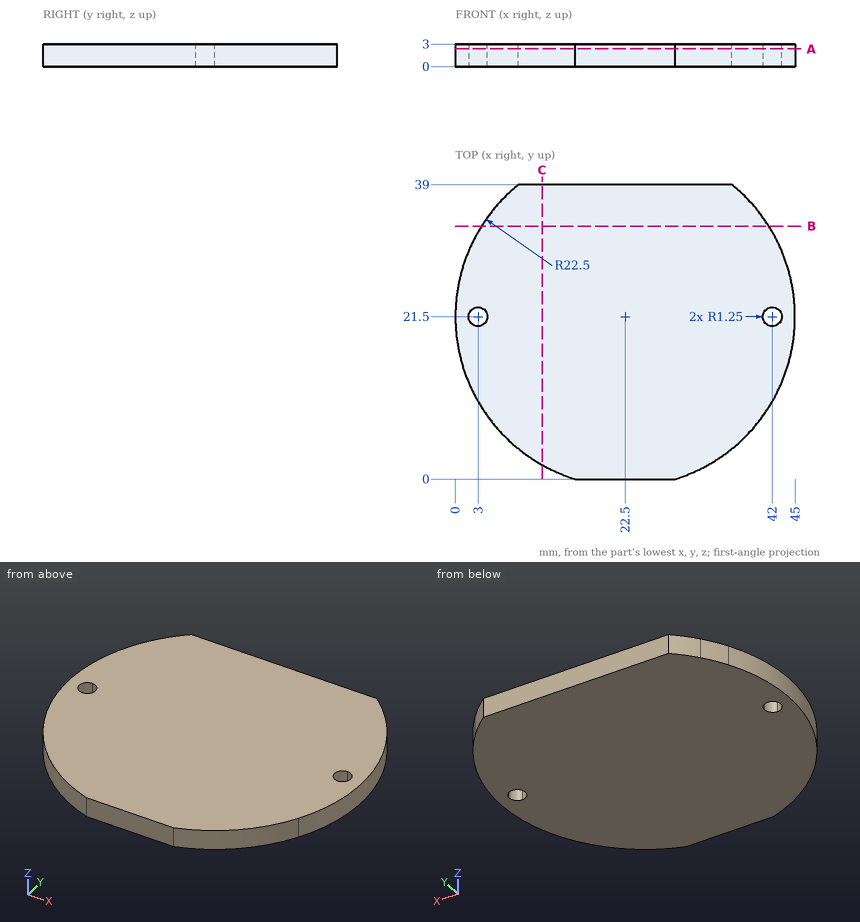
Geometry: see drawing. Coordinates: mm, zero at the bounding-box minimum. Give positions to 0.01 mm unless a question says otherwise; leave off trailing zeros. Order: outer loops, then holes, each group sorted by start corner. A loop starts at its lowest first (then second) coordinate and runs counter-clockwise, first axis right, second up. Notation, with made-up numbers: M -13.5,18.5 L 32.5,18.5 A12 cw 32.5,29.5 Z; hole C 62,13.25 d7. An arc over 180 degrees is marked long. Answer as a JSON object with one key per item and string values.
1. Ray query, line 1 (X direction, y = 21.5, z = 1.95); line 2 (X direction, y = 22.5, z = 1.3); line 3 (Y direction, x = 2, z = 1.4). Return the intervals inside material, ascending. Write a range as [from, to].
Result sheet:
{"line 1": "[0, 1.75], [4.25, 40.75], [43.25, 45]", "line 2": "[0.02, 2.25], [3.75, 41.25], [42.75, 44.98]", "line 3": "[12.23, 20.75], [22.25, 30.77]"}
2. First-contact query: P1, Ø1, axis at y = 31.5, z = 2, coming from the +X side; P2, Ø1.5, axis at y = 22, z = 1.5, coming from the -X side; P3, Ø1, axis at x = 30, z = 1, coming from the -Y side. Flat tips, straight axial feed; report the tip coordinate or a pass-through.
Result sheet:
{"P1": "x = 42.9", "P2": "x = 0", "P3": "y = 0.12"}
3. Cut plane C-C, the plane x = 11.5. Output: boundary loops of the cut face in (y, z), and give its area (3 significant figures).
Result sheet:
{"outline": "M 1.87,0 L 39,0 L 39,3 L 1.87,3 Z", "area": "111 mm²"}
4. Cut plane B-B, the plane y = 33.5. Output: boundary loops of the cut face in (x, z).
Result sheet:
{"outline": "M 3.47,0 L 41.53,0 L 41.53,3 L 3.47,3 Z"}
5. Cut plane A-A, the plane z = 2.35. Output: boundary loops of the cut face in (x, y), and give its area (3 significant figures).
Result sheet:
{"outline": "M 8.36,39 A22.5 ccw 15.87,0 L 29.13,0 A22.5 ccw 36.64,39 Z; hole C 3,21.5 d2.5; hole C 42,21.5 d2.5", "area": "1,480 mm²"}
